Check sheet for the modelled part. Datum: model origin and axes. Units: mm. A direction names the side the tool comes from. Give positions to 0.01 mm unless a question says otherwise; leave off trailing zeros. Loops run counter-clockwise (first coordinate to the right, second up) from the corner with the lowest first, then second, coordinate; pieces in that order, holes last. Notation, with made-up numbers: (53, -5) - (85, -5) arc R21 ccw to (85, 24) - close; hole circle Ø5 at (-17.75, 72.5). An arc over 180 degrees is marked (long way). Answer in a Markdown table with one row per item. Add a question column.
(1) Sectioned sample at A-A on x = 48. Enter the section's corners in (y, z), then the cut area to 3 significant figures.
(2) Draft check along Z on faces 1 (the face through (36.46, 18, -4)), 2 (the face through (23.32, 4, -2)), 3 (the face through (33, 4, -3)). Enter one of: released by +Z, released by -Z, zero draft, split by the parting line, or undercut.
(3) Set-up check for faces 4 (the face through (19.28, 4, -5)), 5 (the face through (0, 5, -3)), 6 (the face through (47, 16, -0.42)): record each of +Z, -Z, +X, -X, +Y, -Y from which the full face is reachable in a straight line by a thin tool's end or side.
(4) Go/stop test with flat-tipped pins: P1, Ø5, axis at x = 30, y = 10.5, coming from the +Z side; P2, Ø1, axis at x = 16.5, z = -0.5, coming from the +Y side; P3, Ø0.8, axis at x = 9.5, y = 2, coming from the -Z side; P4, Ø0.8, axis at y = 3.5, z = -5, coming from the -X side. Record where each tip stops, or that it passes through.
(5) Sectioned sample at C-C on x = 27.5. Enter the section's corners in (y, z), then the cut area to 3 significant figures.
(6) Sectioned sample at B-B on y = 11.25. Enter the section's corners in (x, z), then the cut area to 3 significant figures.
(7) Sectioned sample at D-D on y = 3.5. State how many separate pieces and enclosed holes the cut face has, then the cut area to 3 significant figures.
(8) Thickness scan on L1, parallel to Z at x = 17, y = 2.5; L2, parallel to X at y = 21.5, z = -0.75; L3, parallel to X at y = 13.25, z = -7.5. Record the ranges inside material, lowest first.
from build123d import *

# Parameters (mm, degrees)
SKETCH1_W           = 37.52
SKETCH1_H           = 7.04
SKETCH1_W_2         = 1.5
SKETCH1_H_2         = 1.5
BOSS_EXTRUDE1_DEPTH = 8
SKETCH2_W           = 37.52
SKETCH2_H           = 7.04
BOSS_EXTRUDE2_DEPTH = 2
SKETCH3_W           = 1.06
SKETCH3_H           = 7.04
BOSS_EXTRUDE3_DEPTH = 13
CHAMFER1_SIZE       = 5


with BuildPart() as part:
    # Sketch1 → Boss-Extrude1 (new body)
    with BuildSketch(Plane(origin=(0, 0, 0), x_dir=(1, 0, 0), z_dir=(0, 1, 0))):
        with Locations((18.76, 3.52)):
            Rectangle(SKETCH1_W, SKETCH1_H)
        with Locations((4.79, 2.25)):
            Rectangle(SKETCH1_W_2, SKETCH1_H_2, mode=Mode.SUBTRACT)
        with Locations((2.25, 2.25)):
            Rectangle(SKETCH1_W_2, SKETCH1_H_2, mode=Mode.SUBTRACT)
        with Locations((7.33, 2.25)):
            Rectangle(SKETCH1_W_2, SKETCH1_H_2, mode=Mode.SUBTRACT)
        with Locations((9.87, 2.25)):
            Rectangle(SKETCH1_W_2, SKETCH1_H_2, mode=Mode.SUBTRACT)
        with Locations((12.41, 2.25)):
            Rectangle(SKETCH1_W_2, SKETCH1_H_2, mode=Mode.SUBTRACT)
        with Locations((14.95, 2.25)):
            Rectangle(SKETCH1_W_2, SKETCH1_H_2, mode=Mode.SUBTRACT)
        with Locations((17.49, 2.25)):
            Rectangle(SKETCH1_W_2, SKETCH1_H_2, mode=Mode.SUBTRACT)
        with Locations((20.03, 2.25)):
            Rectangle(SKETCH1_W_2, SKETCH1_H_2, mode=Mode.SUBTRACT)
        with Locations((22.57, 2.25)):
            Rectangle(SKETCH1_W_2, SKETCH1_H_2, mode=Mode.SUBTRACT)
        with Locations((25.11, 2.25)):
            Rectangle(SKETCH1_W_2, SKETCH1_H_2, mode=Mode.SUBTRACT)
        with Locations((27.65, 2.25)):
            Rectangle(SKETCH1_W_2, SKETCH1_H_2, mode=Mode.SUBTRACT)
        with Locations((30.19, 2.25)):
            Rectangle(SKETCH1_W_2, SKETCH1_H_2, mode=Mode.SUBTRACT)
        with Locations((32.73, 2.25)):
            Rectangle(SKETCH1_W_2, SKETCH1_H_2, mode=Mode.SUBTRACT)
        with Locations((35.27, 2.25)):
            Rectangle(SKETCH1_W_2, SKETCH1_H_2, mode=Mode.SUBTRACT)
        with Locations((4.79, 4.79)):
            Rectangle(SKETCH1_W_2, SKETCH1_H_2, mode=Mode.SUBTRACT)
        with Locations((7.33, 4.79)):
            Rectangle(SKETCH1_W_2, SKETCH1_H_2, mode=Mode.SUBTRACT)
        with Locations((9.87, 4.79)):
            Rectangle(SKETCH1_W_2, SKETCH1_H_2, mode=Mode.SUBTRACT)
        with Locations((12.41, 4.79)):
            Rectangle(SKETCH1_W_2, SKETCH1_H_2, mode=Mode.SUBTRACT)
        with Locations((14.95, 4.79)):
            Rectangle(SKETCH1_W_2, SKETCH1_H_2, mode=Mode.SUBTRACT)
        with Locations((17.49, 4.79)):
            Rectangle(SKETCH1_W_2, SKETCH1_H_2, mode=Mode.SUBTRACT)
        with Locations((20.03, 4.79)):
            Rectangle(SKETCH1_W_2, SKETCH1_H_2, mode=Mode.SUBTRACT)
        with Locations((22.57, 4.79)):
            Rectangle(SKETCH1_W_2, SKETCH1_H_2, mode=Mode.SUBTRACT)
        with Locations((25.11, 4.79)):
            Rectangle(SKETCH1_W_2, SKETCH1_H_2, mode=Mode.SUBTRACT)
        with Locations((27.65, 4.79)):
            Rectangle(SKETCH1_W_2, SKETCH1_H_2, mode=Mode.SUBTRACT)
        with Locations((30.19, 4.79)):
            Rectangle(SKETCH1_W_2, SKETCH1_H_2, mode=Mode.SUBTRACT)
        with Locations((32.73, 4.79)):
            Rectangle(SKETCH1_W_2, SKETCH1_H_2, mode=Mode.SUBTRACT)
        with Locations((35.27, 4.79)):
            Rectangle(SKETCH1_W_2, SKETCH1_H_2, mode=Mode.SUBTRACT)
        with Locations((2.25, 4.79)):
            Rectangle(SKETCH1_W_2, SKETCH1_H_2, mode=Mode.SUBTRACT)
    extrude(amount=BOSS_EXTRUDE1_DEPTH)

    # Sketch2 → Boss-Extrude2 (add)
    with BuildSketch(Plane(origin=(0, 8, 0), x_dir=(1, 0, 0), z_dir=(0, 1, 0))):
        with Locations((18.76, 3.52)):
            Rectangle(SKETCH2_W, SKETCH2_H)
    extrude(amount=BOSS_EXTRUDE2_DEPTH)

    # Sketch3 → Boss-Extrude3 (add)
    # profile 1 of 2: a face of its own
    with BuildSketch(Plane(origin=(0, 10, 0), x_dir=(1, 0, 0), z_dir=(0, 1, 0))):
        Polygon((57.96, 9.82), (36.46, 9.82), (36.46, 7.04), (37.52, 7.04), (37.52, 0), (36.46, 0), (36.46, -1.58), (57.96, -1.58), align=None)
        Polygon((38.46, 0.42), (38.46, 6.62), (45.71, 6.62), (45.71, 7.82), (48.71, 7.82), (48.71, 6.62), (55.96, 6.62), (55.96, 0.42), align=None, mode=Mode.SUBTRACT)
    # profile 2 of 2: a face of its own
    with BuildSketch(Plane(origin=(0, 10, 0), x_dir=(1, 0, 0), z_dir=(0, 1, 0))):
        with Locations((36.99, 3.52)):
            Rectangle(SKETCH3_W, SKETCH3_H)
    extrude(amount=BOSS_EXTRUDE3_DEPTH)

    # Chamfer1
    chamfer1_edges = [part.edges().sort_by_distance(p)[0] for p in [
        (36.46, 10, -3.52),
    ]]
    chamfer(chamfer1_edges, length=CHAMFER1_SIZE)


solid = part.part
Reply:
| question | item | result |
|---|---|---|
| 1 | outline | (10, -9.82) - (23, -9.82) - (23, -7.82) - (10, -7.82) - close; (10, -0.42) - (23, -0.42) - (23, 1.58) - (10, 1.58) - close |
| 1 | area | 52.0 mm^2 |
| 2 | face 1 | zero draft |
| 2 | face 2 | undercut |
| 2 | face 3 | undercut |
| 3 | face 4 | -Y |
| 3 | face 5 | +Z, -Z, -X, +Y, -Y |
| 3 | face 6 | +Y, -Y |
| 4 | P1 | z = 0 |
| 4 | P2 | y = 10 |
| 4 | P3 | z = -7.04 |
| 4 | P4 | x = 0 |
| 5 | outline | (0, -7.04) - (10, -7.04) - (10, 0) - (0, 0) - (0, -1.5) - (8, -1.5) - (8, -3) - (0, -3) - (0, -4.04) - (8, -4.04) - (8, -5.54) - (0, -5.54) - close |
| 5 | area | 46.4 mm^2 |
| 6 | outline | (32.71, -7.04) - (36.46, -7.04) - (36.46, -9.82) - (57.96, -9.82) - (57.96, 1.58) - (36.46, 1.58) - (36.46, 0) - (32.71, 0) - close; hole (38.46, -6.62) - (45.71, -6.62) - (45.71, -7.82) - (48.71, -7.82) - (48.71, -6.62) - (55.96, -6.62) - (55.96, -0.42) - (38.46, -0.42) - close |
| 6 | area | 159 mm^2 |
| 7 | separate pieces | 1 |
| 7 | enclosed holes | 28 |
| 7 | area | 201 mm^2 |
| 8 | L1 | -7.04 to -5.54, -4.04 to -3, -1.5 to 0 |
| 8 | L2 | 36.46 to 38.46, 55.96 to 57.96 |
| 8 | L3 | 36.46 to 45.71, 48.71 to 57.96 |
